Can you work these out from the model? Positions are in its coordinate system, mm. A direction names the side the tool comes from. Give positions to 0.01 mm unless a question says otherwise; leave off trailing zeros. Loops run counter-clockwise (first coordinate to the right, second up) from the corner with the lowest first, then second, coordinate; pieces in that order, holes last. Notation, with made-up numbers: (-31.5, 72.5) - (6.5, 72.5) arc R18 ccw to (6.5, 94.5) - close; hole circle Ø7 at (-21.75, 73). An arc over 180 degrees is marked (long way). Write item = value, one per line.
Autodesk Inventor part; units mm, degrees
ref_plane "YZ Plane" through (0, 0, 0) normal (1, 0, 0) x (0, 1, 0)
ref_plane "XZ Plane" through (0, 0, 0) normal (0, 1, 0) x (-1, 0, 0)
ref_plane "XY Plane" through (0, 0, 0) normal (0, 0, 1) x (1, 0, 0)
sketch "スケッチ1" plane through (0, 0, 0) normal (0, 1, 0) x (-1, 0, 0)
  line L0 (27.5, 30) -> (-27.5, 30) construction
  line L1 (-27.5, 30) -> (-27.5, -30) construction
  line L2 (-27.5, -30) -> (27.5, -30) construction
  line L3 (27.5, -30) -> (27.5, 30) construction
  line L4 (27.5, 30) -> (-27.5, -30) construction
  line L5 (-27.5, 30) -> (27.5, -30) construction
  line L6 (27.8, 30.3) -> (-27.8, 30.3)
  line L7 (-27.8, 30.3) -> (-27.8, -30.3)
  line L8 (-27.8, -30.3) -> (27.8, -30.3)
  line L9 (27.8, -30.3) -> (27.8, 30.3)
  line L10 (28.8, 31.3) -> (-28.8, 31.3)
  line L11 (-28.8, 31.3) -> (-28.8, -31.3)
  line L12 (-28.8, -31.3) -> (28.8, -31.3)
  line L13 (28.8, -31.3) -> (28.8, 31.3)
  line L14 (-22.5, 25) -> (22.5, 25) construction
  line L15 (22.5, 25) -> (22.5, -25) construction
  line L16 (22.5, -25) -> (-22.5, -25) construction
  line L17 (-22.5, -25) -> (-22.5, 25) construction
  line L18 (19.5, 30.3) -> (19.5, 25)
  arc A0 (19.5, 25) -> (22.5, 22) centre (22.5, 25) ccw
  line L19 (22.5, 22) -> (27.8, 22)
  line L20 (0, 0) -> (0, 30.3)
  line L21 (0, 30.3) -> (0, 31.3)
  line L22 (0, 0) -> (27.8, 0)
  line L23 (27.8, 0) -> (28.8, 0)
  dimension "d0" = 55
  dimension "d1" = 60
  dimension "d2" = 0.3
  dimension "d3" = 1
  dimension "d4" = 5
  dimension "d5" = 3
extrude "押し出し1" add sketch "スケッチ1" against normal blind 0.8 contours L9 L19 A0 L18 L6 | L6 L21 L10 L13 L23 L9 | L18 A0 L19 L9 L22 L20 L6
extrude "押し出し2" add sketch "スケッチ1" along normal blind 4 contours L9 L19 A0 L18 L6
extrude "押し出し3" add sketch "スケッチ1" along normal blind 5.5 contours L6 L21 L10 L13 L23 L9
hole "穴1" at (22.5, 0, 25) at (-22.5, 0, 25) at (-22.5, 0, -25) at (22.5, 0, -25) direction (0, -1, 0) diameter 2.5 end through all both
fillet "フィレット1" radius 0.5 1 edges at (-22.5, 4, 23.75)
mirror "ミラー1" about plane through (-28.8, 0, 0) normal (0, 0, -1) of "フィレット1", "穴1", "押し出し3", "押し出し2", "押し出し1"
mirror "ミラー2" about plane through (0, 0, 30.3) normal (1, 0, 0) of "フィレット1", "穴1", "押し出し3", "押し出し2", "押し出し1", "ミラー1"
fillet "フィレット2" radius 1 4 edges at (-27.8, 0, 0) (0, 0, 30.3) (27.8, 0, 0) (0, 0, -30.3)
fillet "フィレット3" radius 2 4 edges at (28.8, 2.35, 31.3) (-28.8, 2.35, 31.3) (-28.8, 2.35, -31.3) (28.8, 2.35, -31.3)
properties part number "MD_hf_base_sa_1" material "ABS プラスチック"
Q1. Imagine slicing it at B-B, the plane z = -15. Write out the boundary of the cut face in (x, y), then the cut area to 3 significant figures.
Output:
outline = (-28.8, -0.8) - (28.8, -0.8) - (28.8, 5.5) - (27.8, 5.5) - (27.8, 1) arc R1 cw to (26.8, 0) - (-26.8, 0) arc R1 cw to (-27.8, 1) - (-27.8, 5.5) - (-28.8, 5.5) - close
area = 57.5 mm2
Q2. Which directions (+Z, -Z, +X, -X, +Y, -Y) give clear straight access to the entire face, cutting with the end or side of a thin tool? Please do faces 5 (the flat face through (25, 2, 22)), 6 (the flat face through (0, 2, 31.3)).
Output:
face_5 = +Y
face_6 = +Z, +X, -X, +Y, -Y
Q3. We'd pull the mould along Z, two halves only. Please class faces 1 (the flat face through (-25, 4, -26)), 2 (the cylindrical face through (28.2, 2.39, 30.73)), 3 (the cylindrical face through (28.2, 2.31, -30.73)), 4 (the flat face through (-28, 5.5, 0)): released by +Z, released by -Z, zero draft, split by the parting line, or undercut.
Output:
face_1 = undercut
face_2 = released by +Z
face_3 = released by -Z
face_4 = zero draft
Q4. I need wall thicknesses on L1, parallel to Z at x = -22.5, y = 0.7; L2, parallel to X at y = 2.45, z = 25; L3, parallel to X at y = 4.75, z = -27. Which ranges of each line are inside material? Lowest first, please.
Output:
L1 = -31.3 to -26.25, -23.75 to -22, 22 to 23.75, 26.25 to 31.3
L2 = -28.8 to -23.75, -21.25 to -19.5, 19.5 to 21.25, 23.75 to 28.8
L3 = -28.8 to -27.8, 27.8 to 28.8
Q5. For pin 1 (1 mm diameter, centred on x = -4, z = 5.5, fed in from +Y); pin 2 (4 mm diameter, centred on x = -21.5, z = 28, fed in from +Y); pin 3 (2 mm diameter, centred on x = 22.5, z = -25, fed in from +Y); pin 4 (3 mm diameter, centred on x = -22.5, z = 25, fed in from +Y), each with a flat end and sliding along its axis, tell me the tip position at first contact or that it passes through.
Output:
pin_1 = 0
pin_2 = 4
pin_3 = through
pin_4 = 3.93
Q6. Imagine slicing it at A-A, the plane x = 0.5. Write out the boundary of the cut face in (y, z), then the cut area to 3 significant figures.
Output:
outline = (-0.8, -31.3) - (5.5, -31.3) - (5.5, -30.3) - (1, -30.3) arc R1 cw to (0, -29.3) - (0, 29.3) arc R1 cw to (1, 30.3) - (5.5, 30.3) - (5.5, 31.3) - (-0.8, 31.3) - close
area = 61.5 mm2
